Geometry: final body of the model. Coordinates: model frame, mm. Face numbers are marked on the shaded views. A direction names the side the tool comes from. Give positions to 0.01 mm unless a question says otherwise; leave off trailing zeros. Loops run counter-clockwise (first coordinate to the right, second up) from the corner with the lowest first, then second, coordinate; pieces in that order, holes last. Notation, with made-up numbers: (-26, 87) - (22, 87) arc R17 ccw to (22, 107) - close; hole circle Ø1 at (-3.5, -12.75). An arc over 180 degrees is marked (long way). Answer in a Markdown table with one row per item.
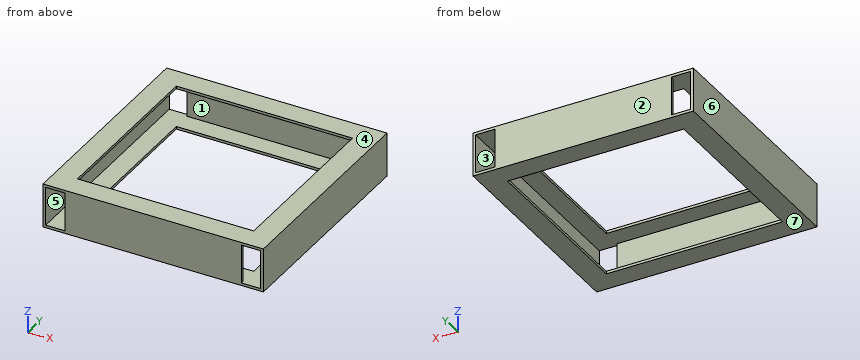
from build123d import *

# Parameters (mm, degrees)
F0_W      = 250
F0_H      = 250
F0_W_2    = 200
F0_H_2    = 200
F1_DEPTH  = 50
F2_W      = 22
F2_H      = 44
F3_DEPTH  = 250
F6_W      = 25
F6_H      = 44
F7_DEPTH  = 125
F8_DEPTH  = 25
F9_DEPTH  = 25
F12_DEPTH = 122
F13_DEPTH = 122


# Not quite as in the source:
# - an extrude ends at something that could not be found from the text; its depth is read off the source's solid
# - a feature of the source that left no trace in its solid (it failed there, or was rolled back) is left out


with BuildPart() as f1:
    # F0 (on Top) → F1 (new body)
    with BuildSketch(Plane.XY):
        Rectangle(F0_W, F0_H)
        Rectangle(F0_W_2, F0_H_2, mode=Mode.SUBTRACT)
    extrude(amount=F1_DEPTH)

    # F2 (on face) → F3 (cut, through all)
    with BuildSketch(Plane.XZ.offset(125)):
        with Locations((-111, 25)):
            Rectangle(F2_W, F2_H)
        with Locations((111, 25)):
            Rectangle(F2_W, F2_H)
    extrude(amount=-F3_DEPTH, mode=Mode.SUBTRACT)

    # F6 (on Right) → F7 (cut, through all)
    with BuildSketch(Plane.YZ):
        with Locations((109.5, 25)):
            Rectangle(F6_W, F6_H)
        with Locations((-109.5, 25)):
            Rectangle(F6_W, F6_H)
    extrude(amount=-F7_DEPTH, mode=Mode.SUBTRACT)

    # F8 (add): a face of the model
    f8_faces = [f1.faces().sort_by_distance(p)[0] for p in [
        (-123.5, 97, 25),
    ]]
    extrude(f8_faces, amount=F8_DEPTH)

    # F9 (add): a face of the model
    f9_faces = [f1.faces().sort_by_distance(p)[0] for p in [
        (-123.5, -122, 25),
    ]]
    extrude(f9_faces, amount=F9_DEPTH)

    # F12 (cut, through all): a face of the model
    f12_faces = [f1.faces().sort_by_distance(p)[0] for p in [
        (0, -111, 25),
    ]]
    extrude(f12_faces, amount=-F12_DEPTH, mode=Mode.SUBTRACT)

    # F13 (cut, through all): a face of the model
    f13_faces = [f1.faces().sort_by_distance(p)[0] for p in [
        (0, 111, 25),
    ]]
    extrude(f13_faces, amount=-F13_DEPTH, mode=Mode.SUBTRACT)


solid = f1.part
Q1. Draft query along Z for the marked faces 4, 5, 6 and 7. Return one class per face: pulls with the +Z half, pulls with the -Z half, needs draft (parallel to the pull), parting line crosses it, or undercut.
Check values:
| item | result |
|---|---|
| face 4 | pulls with the +Z half |
| face 5 | undercut |
| face 6 | needs draft |
| face 7 | pulls with the -Z half |
Q2. Cut plane A-A (z = 8). Output: boundary loops of the cut face in (x, y), and give its area (3 significant figures).
Check values:
| item | result |
|---|---|
| outline | (-125, -125) - (-122, -125) - (-122, 125) - (-125, 125) - close; (-100, -125) - (100, -125) - (100, -122) - (-100, -122) - close; (-100, 122) - (100, 122) - (100, 125) - (-100, 125) - close; (122, -125) - (125, -125) - (125, 125) - (122, 125) - close |
| area | 2,700 mm² |
Q3. Reachability of the marked faces 1, 2 and 3 from +Z, -Z, +X, -X, +Y, -Y: full face, straight path, thin tool, end or side. Return the list, or none.
Check values:
| item | result |
|---|---|
| face 1 | none |
| face 2 | +Z, -Z, +X, -X, +Y |
| face 3 | +Y, -Y |
Q4. Material intervals for line 1 along X through (y, z) = (-93.5, 17); line 2 along X through (y, z) = (13, 2.5), sorted ascending.
Check values:
| item | result |
|---|---|
| line 1 | -125 to -122, 122 to 125 |
| line 2 | -125 to -100, 100 to 125 |
Q5. Cut plane C-C (x = -20.5). Output: boundary loops of the cut face in (y, z).
Check values:
| item | result |
|---|---|
| outline | (-125, 0) - (-100, 0) - (-100, 3) - (-122, 3) - (-122, 47) - (-100, 47) - (-100, 50) - (-125, 50) - close; (100, 0) - (125, 0) - (125, 50) - (100, 50) - (100, 47) - (122, 47) - (122, 3) - (100, 3) - close |
Q6. Cut plane B-B (y = -103.5). Output: boundary loops of the cut face in (x, z), and give its area (3 significant figures).
Check values:
| item | result |
|---|---|
| outline | (-125, 0) - (125, 0) - (125, 50) - (-125, 50) - close; hole (-122, 3) - (122, 3) - (122, 47) - (-122, 47) - close |
| area | 1,760 mm² |
